Read the model definition and answer for the solid it produces. Units are mm, in the model's axes. A direction names the side the tool comes from. Give positions to 0.01 mm unless a question says otherwise; leave off trailing zeros. Loops run counter-clockwise (first coordinate to the right, second up) from the corner with the lowest first, then second, coordinate; pieces in that order, holes last. Notation, with made-up numbers: (32.25, 30.5) - (71.25, 30.5) arc R36 ccw to (71.25, 66.5) - close; hole circle Ø4 at (7, -16). An arc over 180 degrees is marked (long way). Write each question's results on one line, items separated by ' | '. Start each with the question number.
Q1. Find the intervals of material crossed by line 1 (X direction, y = 0, z = -7.6); line 2 (Y direction, x = 54, z = -6.1); line 3 (Z direction, x = 100, y = -7.75), in increasing order. Write a range as from..to.
Q2. The part is cut by section B-B, the plane y = -3.5. Write down the section's boundary in (x, z), plus the area to 3 significant figures.
Q3. The part is cut by section A-A, the plane x = 82. Write down the section's boundary in (y, z), plus the area to 3 significant figures.
Q4. Given pin 1 (2.5 mm diameter, centred on y = -4.5, z = -5, fed in from +X); pin 2 (1.1 mm diameter, centred on x = 56.5, y = -8, fed in from +Z); pin 3 (0.9 mm diameter, centred on x = 70, z = -6.5, fed in from +Y), each flat-ended and moving along its own axis, determine where each tip first touches the part or whether it passes through.
Q5. For faces 5 (the flat face through (-2, -3, -3.557)), 6 (the flat face through (61.62, -9.59, -5.35)), 7 (the flat face through (61.625, -9.616, -6.847)), 8 (the flat face through (123, -6.602, -6)), determine the directions among +Z, -Z, +X, -X, +Y, -Y from which every point of the face is accessible in a straight line to the end or side of a thin tool.
Q6. Determine the mould class of faces 1 (the flat face through (62, -7.602, -6)), 2 (the flat face through (125, -8, -6)), 3 (the flat face through (-5, -5, -6)), 4 (the flat face through (-2, -3, -8.657)) for opening direction X: +X half, -X half, draft (parallel to the pull), parting line (faces both ways), or undercut.
```python
from build123d import *

# Parameters (mm, degrees)
F1_DEPTH = 125
F2_DEPTH = 5
F4_DEPTH = 1
F5_DEPTH = 10


with BuildPart() as f1:
    # F0 (on Right) → F1 (new body)
    with BuildSketch(Plane.YZ):
        Polygon((-8.6018808093, -7.6071059655), (-7.6018808093, -7.6071059655), (-7.6018808093, -4.6071059655), (-8.6018808093, -4.6071059655), (-10.6018808093, -6.1071059655), align=None)
    extrude(amount=F1_DEPTH)

    # F0 (on Right) → F2 (join)
    with BuildSketch(Plane.YZ):
        Polygon((-12.5160943717, -7.2428924032), (-9.1018808093, -8.6571059655), (-6.6018808093, -8.6571059655), (-6.6018808093, -3.5571059655), (-9.1018808093, -3.5571059655), (-12.5160943717, -4.9713195279), (-13.6518808093, -6.1071059655), align=None)
        Polygon((-7.6018808093, -4.6071059655), (-7.6018808093, -7.6071059655), (-8.6018808093, -7.6071059655), (-10.6018808093, -6.1071059655), (-8.6018808093, -4.6071059655), align=None, mode=Mode.SUBTRACT)
        Polygon((-8.6018808093, -7.6071059655), (-7.6018808093, -7.6071059655), (-7.6018808093, -4.6071059655), (-8.6018808093, -4.6071059655), (-10.6018808093, -6.1071059655), align=None)
    extrude(amount=-F2_DEPTH)

    # F3 (on face) → F4 (join)
    with BuildSketch(Plane(origin=(0, -7.6018808093, 0), x_dir=(-1, 0, 0), z_dir=(0, 1, 0))):
        Polygon((-125, -7.1071059655), (-120, -7.1071059655), (-120, -6.1071059655), (-120, -5.1071059655), (-125, -5.1071059655), align=None)
    extrude(amount=F4_DEPTH)

    # F5 (add): a face of the model
    f5_faces = [f1.faces().sort_by_distance(p)[0] for p in [
        (-2.5, -6.6018808093, -6.1071059655),
    ]]
    extrude(f5_faces, amount=F5_DEPTH)


solid = f1.part
```
Check sheet entries:
1) line 1: x = -5..0 | line 2: y = -10.59..-7.6 | line 3: z = -7.61..-4.61
2) outline: (-5, -8.66) - (0, -8.66) - (0, -3.56) - (-5, -3.56) - close | area: 25.5 mm^2
3) outline: (-10.6, -6.11) - (-8.6, -7.61) - (-7.6, -7.61) - (-7.6, -4.61) - (-8.6, -4.61) - close | area: 6.00 mm^2
4) pin 1: stops at x = 0 | pin 2: stops at z = -4.61 | pin 3: stops at y = -7.6
5) face 5: +Z, +X, -X, +Y, -Y | face 6: +Z, +X, -Y | face 7: -Z, +X, -Y | face 8: +Z, -Z, +X, +Y
6) face 1: undercut | face 2: +X half | face 3: -X half | face 4: draft
